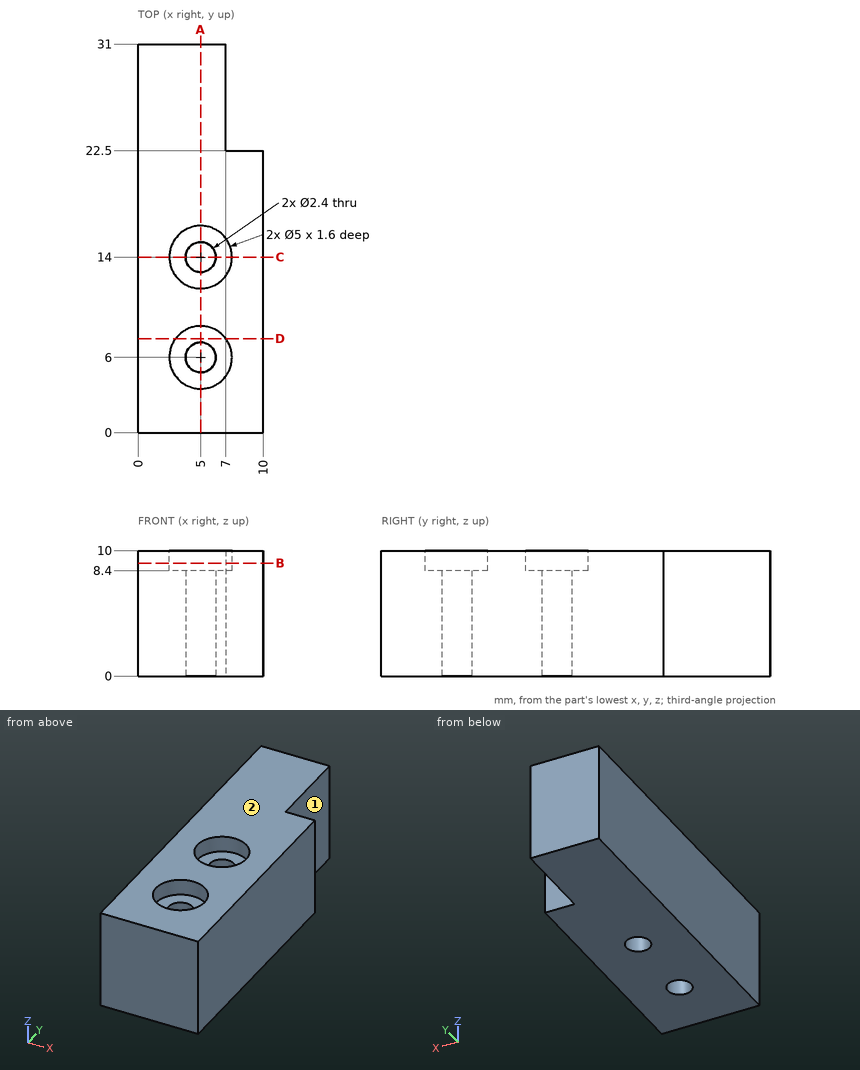
Check sheet for the drawn part. Datum: minimum x, y, z corner. Units: mm. A direction names the side the tool comes from. Coordinates: 2 decimals unless noted, no trailing zeros. Order: outer loops, then holes, each group sorted by start corner. A loop starts at its lowest first (then second) coordinate and runs counter-clockwise, first axis right, second up. Notation, with made-up numbers: (3.5, 9.25) -> (27.5, 9.25) arc R13 ccw to (27.5, 29.25) -> close; hole circle Ø11 at (80.25, -25.5). An arc over 180 degrees is marked (long way). Write each question's results on one line, items separated by ' | '. Start each with the question number.
1) Set-up check for the marked faces 1 and 2: record each of +Z, -Z, +X, -X, +Y, -Y from which the full face is reachable in a straight line by a thin tool's end or side.
2) Depth check by flat-ended pin: pin 1 (3 mm diameter, centred on x = 5, y = 6, fed in from +Z). Enter the tip coordinate at first touch or a pass-through.
3) Material ranges on line 1 along Y through (x, z) = (5, 9.1); line 2 along Y through (x, z) = (5, 7.25); line 3 along Y through (x, z) = (7.75, 6), recorded low to high.
4) Section check A-A (x = 5). Enter the section's corners in (y, z).
5) Section check C-C (y = 14). Enter the section's corners in (x, z).
6) Section check B-B (z = 9). Enter the section's corners in (x, y), and give its area (3 significant figures).
7) Section check D-D (y = 7.5). Enter the section's corners in (x, z), and give its area (3 significant figures).
Checked values:
1) face 1: +Z, -Z, +X, +Y | face 2: +Z, +X, -X, +Y, -Y
2) pin 1: z = 8.4
3) line 1: 0 to 3.5, 8.5 to 11.5, 16.5 to 31 | line 2: 0 to 4.8, 7.2 to 12.8, 15.2 to 31 | line 3: 0 to 22.5
4) outline: (0, 0) -> (4.8, 0) -> (4.8, 8.4) -> (3.5, 8.4) -> (3.5, 10) -> (0, 10) -> close; (7.2, 0) -> (12.8, 0) -> (12.8, 8.4) -> (11.5, 8.4) -> (11.5, 10) -> (8.5, 10) -> (8.5, 8.4) -> (7.2, 8.4) -> close; (15.2, 0) -> (31, 0) -> (31, 10) -> (16.5, 10) -> (16.5, 8.4) -> (15.2, 8.4) -> close
5) outline: (0, 0) -> (3.8, 0) -> (3.8, 8.4) -> (2.5, 8.4) -> (2.5, 10) -> (0, 10) -> close; (6.2, 0) -> (10, 0) -> (10, 10) -> (7.5, 10) -> (7.5, 8.4) -> (6.2, 8.4) -> close
6) outline: (0, 0) -> (10, 0) -> (10, 22.5) -> (7, 22.5) -> (7, 31) -> (0, 31) -> close; hole circle Ø5 at (5, 6); hole circle Ø5 at (5, 14) | area: 245 mm²
7) outline: (0, 0) -> (10, 0) -> (10, 10) -> (7, 10) -> (7, 8.4) -> (3, 8.4) -> (3, 10) -> (0, 10) -> close | area: 93.6 mm²
